```python
from build123d import *

# Parameters (mm, degrees)
SKETCH1_W                                      = 247.65
SKETCH1_H                                      = 10
BOSS_EXTRUDE1_DEPTH                            = 4
CUT_EXTRUDE1_DEPTH                             = 248.732764284
CUT_EXTRUDE2_DEPTH                             = 1.5
CUT_EXTRUDE3_START                             = -114.3
SKETCH13_W                                     = 0.79375
SKETCH13_H                                     = 0.79375
CUT_EXTRUDE3_DEPTH                             = 57.15
LPATTERN1_COUNT                                = 2
LPATTERN1_PITCH                                = 114.3
SKETCH14_W                                     = 20
SKETCH14_H                                     = 4
BOSS_EXTRUDE3_DEPTH                            = 3.5
F_0_80_TAPPED_HOLE2_D                          = 1.19126
CSK_FOR_0_FLAT_HEAD_MACHINE_SCREW1_D           = 1.778
CSK_FOR_0_FLAT_HEAD_MACHINE_SCREW1_CSINK_D     = 3.0226
CSK_FOR_0_FLAT_HEAD_MACHINE_SCREW1_CSINK_ANGLE = 82
MIRROR3_START                                  = -114.3
MIRROR3_COPY_1_SKETCH_W                        = 0.79375
MIRROR3_COPY_1_SKETCH_H                        = 0.79375
MIRROR3_COPY_1_DEPTH                           = 57.15
FILLET6_R                                      = 1.5875


# Read off the part's stored shape, not the designer's step: Cut-Extrude2
with BuildPart() as part:
    # Sketch1 → Boss-Extrude1 (new body)
    with BuildSketch(Plane(origin=(0, 0, 0), x_dir=(1, 0, 0), z_dir=(0, 1, 0))):
        Rectangle(SKETCH1_W, SKETCH1_H)
    extrude(amount=BOSS_EXTRUDE1_DEPTH)

    # Sketch2 → Cut-Extrude1 (cut, through all)
    with BuildSketch(Plane.ZY.offset(123.825)):
        Polygon((-2.05, 1.5), (2.05, 1.5), (2.05, 2), (4.05, 2), (4.05, 4), (-4.05, 4), (-4.05, 2), (-2.05, 2), align=None)
    extrude(amount=-CUT_EXTRUDE1_DEPTH, mode=Mode.SUBTRACT)

    # Cut-Extrude2 outline → Cut-Extrude2 (cut)
    with BuildSketch(Plane(origin=(0, 0, 0), x_dir=(1, 0, 0), z_dir=(0, 1, 0))):
        with BuildLine():
            Line((24.1088, 1.5), (15.1088, 1.5))
            ThreePointArc((15.1088, 1.5), (13.6088, 0), (15.1088, -1.5))
            Line((15.1088, -1.5), (24.1088, -1.5))
            ThreePointArc((24.1088, -1.5), (25.6088, 0), (24.1088, 1.5))
        make_face()
    extrude(amount=CUT_EXTRUDE2_DEPTH, mode=Mode.SUBTRACT)

    # Sketch13 → Cut-Extrude3 (cut)
    with BuildSketch(Plane.ZY.offset(123.825).offset(CUT_EXTRUDE3_START)):
        with Locations((-5, 2)):
            Rectangle(SKETCH13_W, SKETCH13_H)
    cut_extrude3 = extrude(amount=-CUT_EXTRUDE3_DEPTH, mode=Mode.SUBTRACT)

    # LPattern1: Cut-Extrude3 ×2
    with Locations(*[(i * LPATTERN1_PITCH, 0, 0) for i in range(1, LPATTERN1_COUNT)]):
        add(cut_extrude3, mode=Mode.SUBTRACT)

    # Sketch14 → Boss-Extrude3 (add)
    with BuildSketch(Plane(origin=(0, 0, -5), x_dir=(-1, 0, 0), z_dir=(0, 0, -1))):
        with Locations((113.825, 2)):
            Rectangle(SKETCH14_W, SKETCH14_H)
    boss_extrude3 = extrude(amount=BOSS_EXTRUDE3_DEPTH)

    # #0-80 Tapped Hole2 (through all)
    with Locations(Plane(origin=(0, 4, 0), x_dir=(-1, 0, 0), z_dir=(0, 1, 0))):
        with Locations((114.3, -6.9125)):
            f_0_80_tapped_hole2 = Hole(F_0_80_TAPPED_HOLE2_D / 2)

    # CSK for #0 Flat Head Machine Screw1 (through all)
    with Locations(Plane(origin=(0, 4, 0), x_dir=(-1, 0, 0), z_dir=(0, 1, 0))):
        with Locations((105.4125, -6.9125), (122.2375, -6.9125)):
            csk_for_0_flat_head_machine_screw1 = CounterSinkHole(CSK_FOR_0_FLAT_HEAD_MACHINE_SCREW1_D / 2, CSK_FOR_0_FLAT_HEAD_MACHINE_SCREW1_CSINK_D / 2, counter_sink_angle=CSK_FOR_0_FLAT_HEAD_MACHINE_SCREW1_CSINK_ANGLE)

    # Mirror3: Cut-Extrude3, Boss-Extrude3, #0-80 Tapped Hole2, CSK for #0 Flat Head Machine Screw1 across plane
    add(cut_extrude3.mirror(Plane.XY), mode=Mode.SUBTRACT)
    add(boss_extrude3.mirror(Plane.XY))
    add(f_0_80_tapped_hole2.mirror(Plane.XY), mode=Mode.SUBTRACT)
    add(csk_for_0_flat_head_machine_screw1.mirror(Plane.XY), mode=Mode.SUBTRACT)

    # Mirror3 copy 1 sketch → Mirror3 copy 1 (cut)
    with BuildSketch(Plane(origin=(-9.525, 0, 0), x_dir=(0, 0, -1), z_dir=(-1, 0, 0)).offset(MIRROR3_START)):
        with Locations((-5, -2)):
            Rectangle(MIRROR3_COPY_1_SKETCH_W, MIRROR3_COPY_1_SKETCH_H)
    extrude(amount=-MIRROR3_COPY_1_DEPTH, mode=Mode.SUBTRACT)

    # Fillet6
    fillet6_edges = [part.edges().sort_by_distance(p)[0] for p in [
        (-103.825, 2, -5),
        (-103.825, 2, 5),
    ]]
    fillet(fillet6_edges, radius=FILLET6_R)


solid = part.part
```
CAD build for the part. Positions are in the model's coordinates, mm. A direction names the side the tool comes from. Round coordinates to 2 decimals unless told otherwise and drop trailing zeros. Order: outer loops, then holes, each group sorted by start corner. A loop starts at its lowest first (then second) coordinate and runs counter-clockwise, first axis right, second up.
Q1. Slice it at A-A (x = 8). Write the cut outline in (y, z).
Q2. Two-plate mould, pull along Z, no slides. Class faces 1 (the flat face through (9, 3, -5)), 2 (the flat face through (-2, 1.5, 0)), 3 (the flat face through (-123.825, 1, 0)): pulls with the +Z half, pulls with the -Z half, needs draft (parallel to the pull), parting line crosses it, or undercut.
Q3. Slice it at B-B (y = 0.9). Write the cut outline in (x, z) (1 decimal), and give its area (3 significant figures).
Q4. Drop flat-ended pins along their axis: pin 1 (2 mm diameter, centred on x = -37.5, y = 3, fed in from +Z); pin 2 (1.2 mm diameter, centred on x = 39.5, y = 2, fed in from -Z); pin 3 (0.6 mm diameter, centred on y = 1.5, z = 7, fed in from +X) (3 decimals). Give the stop position or say it passes through.
Q5. Which spindle directions (+Z, -Z, +X, -X, +Y, -Y) get a long thin tool onto all of the face, cutting with end or side? Do faces 4 (the flat face through (9, 3, 5)), 5 (the flat face through (-114, 2, -8.5)). Say none if no direction does.
Q6. Wall check: L1, parallel to Z at x = -114.3, y = 1.95; L2, parallel to X at y = 0.9, z = -7 (3 decimals); L3, parallel to Z at x = -66, y = 2.9. Give the ranges that are in metal, low to high.
Q7. Slice it at C-C (x = 62). Write the cut outline in (y, z), and give its area (4 significant figures).
Results below:
1. outline: (0, -5) - (1.6, -5) - (1.6, -4.6) - (2.4, -4.6) - (2.4, -5) - (4, -5) - (4, -4.05) - (2, -4.05) - (2, -2.05) - (1.5, -2.05) - (1.5, 2.05) - (2, 2.05) - (2, 4.05) - (4, 4.05) - (4, 5) - (2.4, 5) - (2.4, 4.6) - (1.6, 4.6) - (1.6, 5) - (0, 5) - close
2. face 1: pulls with the -Z half
2. face 2: undercut
2. face 3: needs draft
3. outline: (-123.8, -8.5) - (-103.8, -8.5) - (-103.8, -6.6) arc R1.6 cw to (-102.2, -5) - (123.8, -5) - (123.8, 5) - (-102.2, 5) arc R1.6 cw to (-103.8, 6.6) - (-103.8, 8.5) - (-123.8, 8.5) - close; hole circle Ø1.8 at (-122.2, -6.9); hole circle Ø1.8 at (-122.2, 6.9); hole circle Ø1.2 at (-114.3, -6.9); hole circle Ø1.2 at (-114.3, 6.9); hole circle Ø1.8 at (-105.4, -6.9); hole circle Ø1.8 at (-105.4, 6.9); hole (15.1, -1.5) - (24.1, -1.5) arc R1.5 ccw to (24.1, 1.5) - (15.1, 1.5) arc R1.5 ccw to start
3. area: 2,570 mm2
4. pin 1: stops at z = 5
4. pin 2: stops at z = -5
4. pin 3: stops at x = -103.825
5. face 4: +Z, +X, +Y, -Y
5. face 5: -Z, +X, -X, +Y, -Y
6. L1: z = -8.5 to -7.51, -6.32 to -2.05, 2.05 to 6.32, 7.51 to 8.5
6. L2: x = -123.825 to -123.122, -121.353 to -114.889, -113.711 to -106.297, -104.528 to -103.825
6. L3: z = -5 to -4.05, 4.05 to 5
7. outline: (0, -5) - (4, -5) - (4, -4.05) - (2, -4.05) - (2, -2.05) - (1.5, -2.05) - (1.5, 2.05) - (2, 2.05) - (2, 4.05) - (4, 4.05) - (4, 5) - (0, 5) - close
7. area: 21.75 mm2
